```python
from build123d import *

# Parameters (mm, degrees)
SZKIC1_R                    = 12.5
DODANIE_WYCI_GNI_CIE2_DEPTH = 15
SZKIC3_R                    = 8.5
DODANIE_WYCI_GNI_CIE3_DEPTH = 15
DODANIE_WYCI_GNI_CIE4_DEPTH = 7.5
OTWORY_USTALAJ_CE_8_0MM1_D  = 8
OTWORY_USTALAJ_CE_3_0MM2_D  = 3


with BuildPart() as part:
    # Szkic1 → Dodanie-wyci_gni_cie2 (new body)
    with BuildSketch(Plane(origin=(0, 0, 0), x_dir=(1, 0, 0), z_dir=(0, 1, 0))):
        with Locations(Location((0, 0, 0), (0, 0, 270))):
            Circle(SZKIC1_R)
    extrude(amount=DODANIE_WYCI_GNI_CIE2_DEPTH)



with BuildPart() as body_2:
    # Szkic3 → Dodanie-wyci_gni_cie3 (new body)
    with BuildSketch(Plane(origin=(0, 0, 0), x_dir=(1, 0, 0), z_dir=(0, 1, 0))):
        with Locations(Location((35, 0, 0), (0, 0, 270))):
            Circle(SZKIC3_R)
    extrude(amount=DODANIE_WYCI_GNI_CIE3_DEPTH)


with BuildPart() as part_1:
    add(part.part)

    add(body_2.part)  # Dodanie-wyci_gni_cie4 merges body 2
    # Szkic4 → Dodanie-wyci_gni_cie4 (add)
    with BuildSketch(Plane(origin=(0, 0, 0), x_dir=(-1, 0, 0), z_dir=(0, -1, 0))):
        with BuildLine():
            ThreePointArc((-6.778939078, 10.502189533), (-12.5, 0), (-6.778939078, -10.502189533))
            add(Edge.make_bspline(
                [(-6.778939078, -10.502189533), (-20.225507154, -7.239536671), (-33.411274741, -8.350206707)],
                knots=[0, 0, 0, 0.631379274, 0.631379274, 0.631379274], degree=2))
            ThreePointArc((-33.411274741, -8.350206707), (-26.503236916, -0.234557237), (-32.953022418, 8.249841379))
            add(Edge.make_bspline(
                [(-6.778939078, 10.502189533), (-20.078070114, 6.877362512), (-32.953022418, 8.249841379)],
                knots=[0, 0, 0, 0.617827196, 0.617827196, 0.617827196], degree=2))
        make_face()
    extrude(amount=-DODANIE_WYCI_GNI_CIE4_DEPTH)

    # Otwory ustalaj_ce _8.0mm1 (through all)
    with Locations(Plane(origin=(0, 15, 0), x_dir=(1, 0, 0), z_dir=(0, 1, 0))):
        with Locations((0, 0)):
            Hole(OTWORY_USTALAJ_CE_8_0MM1_D / 2)

    # Otwory ustalaj_ce _3.0mm2 (through all)
    with Locations(Plane(origin=(0, 15, 0), x_dir=(1, 0, 0), z_dir=(0, 1, 0))):
        with Locations((35, 0)):
            Hole(OTWORY_USTALAJ_CE_3_0MM2_D / 2)


solid = part_1.part
```
The listing builds one solid part. Answer for the finished solid, in the listing's coordinates (mm). A direction names the side the tool comes from. Round coordinates to 2 decimals unless told otherwise and drop trailing zeros. Order: outer loops, then holes, each group sorted by start corner. A loop starts at its lowest first (then second) coordinate and runs counter-clockwise, first axis right, second up. Notation, with made-up numbers: (-26, 37.5) -> (24, 37.5) arc R25 cw to (24, 69.5) -> close; hole circle Ø9 at (-7, -40). An arc over 180 degrees is marked (long way). Answer as CSV lines item,"result".
Q1. Given pin 1 (2 mm diameter, centred on y = 10, z = 7.5, fed in from +X); pin 2 (6 mm diameter, centred on x = 28, y = 3, fed in from -Z); pin 3 (5 mm diameter, centred on y = 2, z = 3, fed in from +X), each flat-ended and moving along its own axis, determine where each tip first touches the part or whether it passes through.
Computed values:
pin 1,"stops at x = 40.48"
pin 2,"stops at z = -8.07"
pin 3,"stops at x = 43.49"
Q2. A cutting plane is placed at C-C on y = 11.25. Determine the outline of the cut face in (x, z).
Computed values:
outline,"circle Ø25 at (0, 0); circle Ø17 at (35, 0); hole circle Ø8 at (0, 0); hole circle Ø3 at (35, 0)"
Q3. A cutting plane is placed at D-D on x = 0. Determine the outline of the cut face in (y, z), plus the area to 3 significant figures.
Computed values:
outline,"(0, -12.5) -> (15, -12.5) -> (15, -4) -> (0, -4) -> close; (0, 4) -> (15, 4) -> (15, 12.5) -> (0, 12.5) -> close"
area,"255 mm^2"
Q4. A cutting plane is placed at A-A on z = 0. Determine the outline of the cut face in (x, y), plus the area to 3 significant figures.
Computed values:
outline,"(-12.5, 0) -> (-4, 0) -> (-4, 15) -> (-12.5, 15) -> close; (4, 0) -> (33.5, 0) -> (33.5, 15) -> (26.5, 15) -> (26.5, 7.5) -> (12.5, 7.5) -> (12.5, 15) -> (4, 15) -> close; (36.5, 0) -> (43.5, 0) -> (43.5, 15) -> (36.5, 15) -> close"
area,"570 mm^2"
Q5. For a pull along Z with two mould halves and no side action, classify faces 3 (the flat face through (35, 15, 2)), 4 (the cylindrical face through (36.2, 7.4, 0.9)), 5 (the cylindrical face through (0.867, 7.395, 3.905)), 6 (the cylindrical face through (-11.09, 7.4, 5.77)) as +Z half, -Z half, draft (parallel to the pull), parting line (faces both ways), or undercut.
Computed values:
face 3,"draft"
face 4,"undercut"
face 5,"undercut"
face 6,"parting line"
Q6. A cutting plane is placed at B-B on x = 35. Determine the outline of the cut face in (y, z).
Computed values:
outline,"(0, -8.5) -> (15, -8.5) -> (15, -1.5) -> (0, -1.5) -> close; (0, 1.5) -> (15, 1.5) -> (15, 8.5) -> (0, 8.5) -> close"
Q7. Which of the six approach directions +Z, -Z, +X, -X, +Y, -Y give full straight-line access (tool end or side, diameter ignored) to faces 1 (the cylindrical face through (43.428, 9.062, -1.107)), 2 (the flat face through (16, 0, 0))?
Computed values:
face 1,"+Y"
face 2,"+Z, -Z, +X, -X, -Y"
Q8. Consider line 1 (Z direction, x = 0, y = 0.75); line 2 (Z direction, x = 35, y = 3); line 3 (Y direction, x = 27.5, z = -7.5). Determine where each line is inside the solid, lowest interval first. Write a range as from..to.
Computed values:
line 1,"z = -12.5..-4, 4..12.5"
line 2,"z = -8.5..-1.5, 1.5..8.5"
line 3,"y = 0..7.5"
